from build123d import *

# Parameters (mm, degrees)
SKETCH_1_W      = 15
SKETCH_1_H      = 25
EXTRUDE_1_DEPTH = 1
M3X0_5_1_D      = 2.5
M3X0_5_1_DEPTH  = 8.5
M3X0_5_1_TIP    = 0.751075774
SKETCH_4_W      = 15
SKETCH_4_H      = 1
EXTRUDE_2_DEPTH = 20
M3X0_5_2_D      = 2.5
M3X0_5_2_DEPTH  = 8.5
M3X0_5_2_TIP    = 0.751075774


with BuildPart() as part:
    # ｽｹｯﾁ1 → ﾎﾞｽ - 押し出し1 (new body)
    with BuildSketch(Plane.XY):
        with Locations((7.5, 12.5)):
            Rectangle(SKETCH_1_W, SKETCH_1_H)
    extrude(amount=EXTRUDE_1_DEPTH)

    # M3x0.5 ねじ穴1
    with Locations(Plane(origin=(0, 0, 0), x_dir=(-1, 0, 0), z_dir=(0, 0, -1))):
        with Locations((-12.5, 11), (-12.5, 4)):
            Hole(M3X0_5_1_D / 2, depth=M3X0_5_1_DEPTH)
            with Locations((0, 0, -(M3X0_5_1_DEPTH + M3X0_5_1_TIP / 2))):  # 118° drill point
                Cone(0, M3X0_5_1_D / 2, M3X0_5_1_TIP, mode=Mode.SUBTRACT)

    # ｽｹｯﾁ4 → ﾎﾞｽ - 押し出し2 (add)
    with BuildSketch(Plane(origin=(0, 0, 0), x_dir=(-1, 0, 0), z_dir=(0, 0, -1))):
        with Locations((-7.5, 24.5)):
            Rectangle(SKETCH_4_W, SKETCH_4_H)
    extrude(amount=EXTRUDE_2_DEPTH)

    # M3x0.5 ねじ穴2
    with Locations(Plane(origin=(0, 24, 0), x_dir=(-1, 0, 0), z_dir=(0, -1, 0))):
        with Locations((-8, 5.010585189), (-7.540008994, 15)):
            Hole(M3X0_5_2_D / 2, depth=M3X0_5_2_DEPTH)
            with Locations((0, 0, -(M3X0_5_2_DEPTH + M3X0_5_2_TIP / 2))):  # 118° drill point
                Cone(0, M3X0_5_2_D / 2, M3X0_5_2_TIP, mode=Mode.SUBTRACT)


solid = part.part
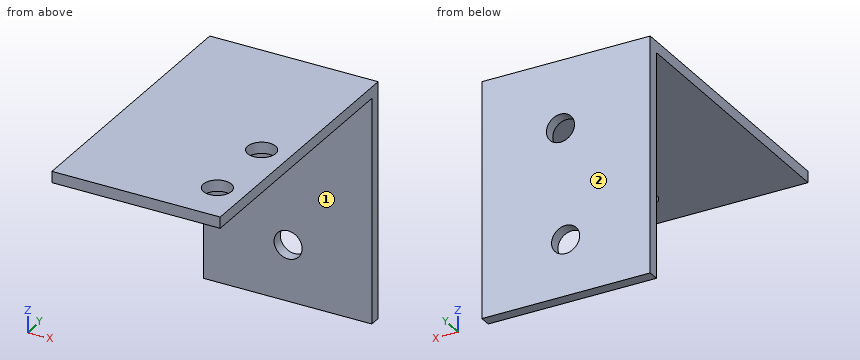
For this review, take the finished solid that the model builds, in its own axes (mm). Face numbers are marked on the shaded views. A direction names the side the tool comes from. Round coordinates to 2 decimals unless told otherwise and drop trailing zeros. Write each loop counter-clockwise with the first axis right and the second up, starting at its lowest first coordinate (ties: lowest second). Pieces come first, ordered by that corner, then holes. Notation, with made-up numbers: M 60.25,78 L 113.25,78 A8 cw 113.25,84 Z; hole C 24,-4.75 d3. An arc over 180 degrees is marked long. Write item = value, one per line. Start each with the question number.
(1) Clearance check with flat-ended pins moving along their axes: pin 1 Ø4 at (x, z) = (6, -13) entering from -Y; pin 2 Ø3 at (x, y) = (12.5, 11) entering from -Z. State where each tip first meets the part, or that it passes through.
(2) For line 1 along Y through (x, z) = (12.5, 0.6); line 2 along X through (y, z) = (24.4, -15); line 3 along Z through (x, y) = (9.5, 14.5), list the stretches that pass through material, from the lowest coordinate up.
(3) We need section B-B (x = 12.5). Give the boundary of the cut face in (y, z).
(4) For the marked faces 1 and 2, list the 3-axis set-ups (+Z, -Z, +X, -X, +Y, -Y) from which the entire face can be reached by the end or side of a thin tool; tool diameter is ignored.
(5) We need section A-A (z = -15). Give the boundary of the cut face in (x, y).
(6) We need section C-C (y = 4). Give the boundary of the cut face in (x, z), then the cut area to 3 significant figures.
(7) We need section D-D (x = 3.5). Give the boundary of the cut face in (y, z).
Results found:
q1.pin_1 = 24
q1.pin_2 = 0
q2.line_1 = 0 to 2.75, 5.25 to 9.75, 12.25 to 25
q2.line_2 = 0 to 6.29, 8.79 to 15
q2.line_3 = 0 to 1
q3.outline = M 0,0 L 2.75,0 L 2.75,1 L 0,1 Z; M 5.25,0 L 9.75,0 L 9.75,1 L 5.25,1 Z; M 12.25,0 L 24,0 L 24,-20 L 25,-20 L 25,1 L 12.25,1 Z
q4.face_1 = -Z, +X, -X, -Y
q4.face_2 = +Z, -Z, +X, -X, +Y
q5.outline = M 0,24 L 6.29,24 L 6.29,25 L 0,25 Z; M 8.79,24 L 15,24 L 15,25 L 8.79,25 Z
q6.outline = M 0,0 L 11.25,0 L 11.25,1 L 0,1 Z; M 13.75,0 L 15,0 L 15,1 L 13.75,1 Z
q6.area = 12.5 mm²
q7.outline = M 0,0 L 24,0 L 24,-20 L 25,-20 L 25,1 L 0,1 Z
